```python
from build123d import *

# Parameters (mm, degrees)
SKETCH_1_W          = 4
SKETCH_1_H          = 4
SKETCH_1_H_2        = 15
EXTRUDE_1_DEPTH     = 23
EXTRUDE_2_DEPTH     = 4
SKETCH_3_R          = 6
CUT_EXTRUDE_1_DEPTH = 36.5
SKETCH_4_R          = 4
CUT_EXTRUDE_2_DEPTH = 4


with BuildPart() as part:
    # Эскиз1 → Бобышка-Вытянуть1 (new body)
    with BuildSketch(Plane(origin=(0, 0, 0), x_dir=(1, 0, 0), z_dir=(0, 1, 0))):
        Polygon((22.5, 10.5), (-22.5, 10.5), (-22.5, 4.5), (-14.5, 4.5), (-10.5, 4.5), (12.5, 4.5), (16.5, 4.5), (22.5, 4.5), align=None)
        with Locations((-12.5, 2.5)):
            Rectangle(SKETCH_1_W, SKETCH_1_H)
        with Locations((14.5, -3)):
            Rectangle(SKETCH_1_W, SKETCH_1_H_2)
    extrude(amount=EXTRUDE_1_DEPTH)

    # Эскиз2 → Бобышка-Вытянуть2 (add)
    with BuildSketch(Plane(origin=(0, 23, 0), x_dir=(1, 0, 0), z_dir=(0, 1, 0))):
        Polygon((12.5, -10.5), (-2.5, 4.5), (12.5, 4.5), align=None)
    extrude(amount=-EXTRUDE_2_DEPTH)

    # Эскиз3 → Вырез-Вытянуть1 (cut, through all)
    with BuildSketch(Plane.XY.offset(-4.5)):
        with Locations((1, 11.5)):
            Circle(SKETCH_3_R)
    extrude(amount=-CUT_EXTRUDE_1_DEPTH, mode=Mode.SUBTRACT)

    # Эскиз4 → Вырез-Вытянуть2 (cut)
    with BuildSketch(Plane.ZY.offset(-16.5)):
        with Locations(Location((3, 11.5, 0), (0, 0, 180))):
            Circle(SKETCH_4_R)
    extrude(amount=CUT_EXTRUDE_2_DEPTH, mode=Mode.SUBTRACT)


solid = part.part
```
Geometry: final body of the model. Coordinates: model frame, mm. A direction names the side the tool comes from. Coordinates: 2 decimals unless noted, no trailing zeros. Loops run counter-clockwise (first coordinate to the right, second up) from the corner with the lowest first, then second, coordinate; pieces in that order, holes last. Notation, with made-up numbers: (11, 78) -> (39, 78) arc R24 ccw to (39, 102) -> close; hole circle Ø3 at (37.5, 1.5). An arc over 180 degrees is marked (long way). Use a Markdown table: item, result. Add a question column.
(1) Pin query (flat end, axial travel): pin 1 Ø9.5 at (x, y) = (1, 11.5) entering from +Z; pin 2 Ø4.5 at (y, z) = (14.5, 6) entering from +X; pin 3 Ø6.5 at (x, y) = (-18.5, 16) entering from +Z; pin 4 Ø1.2 at (x, y) = (-13.5, 9.5) entering from +Z. Return the tip coordinate at first contact, or that it passes through.
(2) Line query: line 1 along Y through (x, z) = (1, -7.15); line 2 along X through (y, z) = (15.25, -3.5); line 3 along Z through (x, y) = (-6.5, 8.5). Output: solid intervals per line, ascending.
(3) Section query A-A, the plane y = 11.5. Return loops of the section in (x, z), plus the area to 3 significant figures.
(4) Section query D-D, the plane z = -6.75. Return loops of the section in (x, y).
(5) Section query C-C, the plane z = 3. Return loops of the section in (x, y), plus the area to 3 significant figures.
(6) Access query for faces 5 (the flat face through (16.5, 8.8, -0.2)), 6 (the flat face through (12.5, 7, 3)), 7 (the flat face through (-10.5, 11, -2)), 8 (the flat face through (-13, 11, -0.5)), 9 (the cylindrical face through (14.528, 15.405, 3.867)). Directions: +Z, -Z, +X, -X, +Y, -Y. A direction counts if a zero-diameter tool reaches every point of the face in a straight line with its end or side. Return the directions, or none.
(7) Mould query, pull axis X, two halves, no side actions, for faces 1 (the flat face through (22.5, 11, -7)), 2 (the flat face through (5, 23, -5)), 3 (the flat face through (5, 21, 3)), 4 (the flat face through (-22.5, 11, -8)). Classes: pulls with the +X half, pulls with the -X half, needs draft (parallel to the pull), parting line crosses it, or undercut.
(8) Section query B-B, the plane x = 1. Return loops of the section in (y, z).
Answer:
| question | item | result |
|---|---|---|
| 1 | pin 1 | passes through |
| 1 | pin 2 | stops at x = 16.5 |
| 1 | pin 3 | stops at z = -4.5 |
| 1 | pin 4 | stops at z = -0.5 |
| 2 | line 1 | y = 0 to 5.5, 17.5 to 23 |
| 2 | line 2 | x = -14.5 to -10.5, 12.5 to 16.5 |
| 2 | line 3 | z = -10.5 to -4.5 |
| 3 | outline | (-22.5, -10.5) -> (-5, -10.5) -> (-5, -4.5) -> (-10.5, -4.5) -> (-10.5, -0.5) -> (-14.5, -0.5) -> (-14.5, -4.5) -> (-22.5, -4.5) -> close; (7, -10.5) -> (22.5, -10.5) -> (22.5, -4.5) -> (16.5, -4.5) -> (16.5, -1) -> (12.5, -1) -> (12.5, -4.5) -> (7, -4.5) -> close; (12.5, 7) -> (16.5, 7) -> (16.5, 10.5) -> (12.5, 10.5) -> close |
| 3 | area | 242 mm^2 |
| 4 | outline | (-22.5, 0) -> (22.5, 0) -> (22.5, 23) -> (-22.5, 23) -> close; hole circle Ø12 at (1, 11.5) |
| 5 | outline | (5, 19) -> (12.5, 19) -> (12.5, 15.5) -> (16.5, 15.5) -> (16.5, 23) -> (5, 23) -> close; (12.5, 0) -> (16.5, 0) -> (16.5, 7.5) -> (12.5, 7.5) -> close |
| 5 | area | 90.0 mm^2 |
| 6 | face 5 | +Z, +X, +Y, -Y |
| 6 | face 6 | +Z, -Y |
| 6 | face 7 | +Z, +Y, -Y |
| 6 | face 8 | +Z, -X, +Y, -Y |
| 6 | face 9 | +X |
| 7 | face 1 | pulls with the +X half |
| 7 | face 2 | needs draft |
| 7 | face 3 | undercut |
| 7 | face 4 | pulls with the -X half |
| 8 | outline | (0, -10.5) -> (5.5, -10.5) -> (5.5, -4.5) -> (0, -4.5) -> close; (17.5, -10.5) -> (23, -10.5) -> (23, -1) -> (19, -1) -> (19, -4.5) -> (17.5, -4.5) -> close |
